Verification items for the finished model (mm, model axes). Give positions to 0.01 mm unless a question says otherwise; leave off trailing zeros. Order: outer loops, then holes, each group sorted by start corner. A loop starts at its lowest first (then second) coordinate and runs counter-clockwise, first axis right, second up.
(1) Scan lines: L1, parallel to Y at x = 102, z = 6 (3 decimals); L2, parallel to Y at x = 65, z = 2.25; L3, parallel to X at y = 166, z = 5.25 (3 decimals). Record each from-to range of solid material in increasing order.
(2) Sectioned sample at C-C on z = 3. Count the separate pieces of the cut face and the enclosed holes in it, plus the area to 3 significant figures.
(3) Sectioned sample at A-A on y = 185. Record the cut outline in (x, z).
(4) Gauge pin test, flat ends, axial feed: pin 1 (2 mm diameter, centred on y = 22.5, z = 3, fed in from +X); pin 2 (3 mm diameter, centred on x = -2.5, z = 2, fed in from -Y); pin 3 (1.5 mm diameter, centred on y = 225.5, z = 1.5, fed in from -X). Record the tip position at first contact, or that the pin passes through.
```python
from build123d import *

# Parameters (mm, degrees)
SKETCH2_W           = 6.096
SKETCH2_H           = 19.230769231
SKETCH2_W_2         = 19.230769231
SKETCH2_H_2         = 6.096
SKETCH2_W_3         = 19.23076923
SKETCH2_H_3         = 19.23076923
BOSS_EXTRUDE2_DEPTH = 6.096
SKETCH3_R           = 5
CUT_EXTRUDE1_DEPTH  = 363.225735762


with BuildPart() as part:
    # Sketch2 → Boss-Extrude2 (new body)
    # profile 1 of 29: a face of its own
    with BuildSketch(Plane.XY):
        Polygon((0, 19.230769231), (0, 0), (19.230769231, 0), (38.461538462, 0), (57.692307692, 0), (76.923076923, 0), (96.153846154, 0), (115.384615385, 0), (134.615384615, 0), (153.846153846, 0), (173.076923077, 0), (192.307692308, 0), (211.538461538, 0), (230.769230769, 0), (250, 0), (250, 19.230769231), (250, 38.461538462), (250, 57.692307692), (250, 76.923076923), (250, 96.153846154), (250, 115.384615385), (250, 134.615384615), (250, 153.846153846), (250, 173.076923077), (250, 192.307692308), (250, 211.538461538), (250, 230.769230769), (250, 250), (230.769230769, 250), (211.538461538, 250), (192.307692308, 250), (173.076923077, 250), (153.846153846, 250), (134.615384615, 250), (115.384615385, 250), (96.153846154, 250), (76.923076923, 250), (57.692307692, 250), (38.461538462, 250), (19.230769231, 250), (0, 250), (0, 230.769230769), (0, 211.538461538), (0, 192.307692308), (0, 173.076923077), (0, 153.846153846), (0, 134.615384615), (0, 115.384615385), (0, 96.153846154), (0, 76.923076923), (0, 57.692307692), (0, 38.461538462), align=None)
        Polygon((80.825, 104), (80.825, 80.825), (104, 80.825), (104, 77.65), (80.825, 77.65), (79.825, 77.65), (79.825, 80.825), (77.65, 80.825), (77.65, 104), align=None, mode=Mode.SUBTRACT)
        Polygon((146, 80.825), (169.175, 80.825), (169.175, 104), (172.35, 104), (172.35, 80.825), (170.175, 80.825), (170.175, 77.65), (169.175, 77.65), (146, 77.65), align=None, mode=Mode.SUBTRACT)
        Polygon((104, 169.175), (80.825, 169.175), (80.825, 146), (77.65, 146), (77.65, 169.175), (79.825, 169.175), (79.825, 172.35), (80.825, 172.35), (104, 172.35), align=None, mode=Mode.SUBTRACT)
        Polygon((169.175, 146), (169.175, 169.175), (146, 169.175), (146, 172.35), (169.175, 172.35), (170.175, 172.35), (170.175, 169.175), (172.35, 169.175), (172.35, 146), align=None, mode=Mode.SUBTRACT)
    # profile 2 of 29: a face of its own
    with BuildSketch(Plane.XY):
        with Locations((-3.048, 9.615384616)):
            Rectangle(SKETCH2_W, SKETCH2_H)
    # profile 3 of 29: a face of its own
    with BuildSketch(Plane.XY):
        with Locations((9.615384616, -3.048)):
            Rectangle(SKETCH2_W_2, SKETCH2_H_2)
    # profile 4 of 29: a face of its own
    with BuildSketch(Plane.XY):
        with Locations((48.076923077, -3.048)):
            Rectangle(SKETCH2_W_3, SKETCH2_H_2)
    # profile 5 of 29: a face of its own
    with BuildSketch(Plane.XY):
        with Locations((-3.048, 48.076923077)):
            Rectangle(SKETCH2_W, SKETCH2_H_3)
    # profile 6 of 29: a face of its own
    with BuildSketch(Plane.XY):
        with Locations((86.538461539, -3.048)):
            Rectangle(SKETCH2_W_2, SKETCH2_H_2)
    # profile 7 of 29: a face of its own
    with BuildSketch(Plane.XY):
        with Locations((-3.048, 86.538461539)):
            Rectangle(SKETCH2_W, SKETCH2_H)
    # profile 8 of 29: a face of its own
    with BuildSketch(Plane.XY):
        with Locations((125, -3.048)):
            Rectangle(SKETCH2_W_3, SKETCH2_H_2)
    # profile 9 of 29: a face of its own
    with BuildSketch(Plane.XY):
        with Locations((-3.048, 125)):
            Rectangle(SKETCH2_W, SKETCH2_H_3)
    # profile 10 of 29: a face of its own
    with BuildSketch(Plane.XY):
        with Locations((163.461538462, -3.048)):
            Rectangle(SKETCH2_W_2, SKETCH2_H_2)
    # profile 11 of 29: a face of its own
    with BuildSketch(Plane.XY):
        with Locations((-3.048, 163.461538462)):
            Rectangle(SKETCH2_W, SKETCH2_H)
    # profile 12 of 29: a face of its own
    with BuildSketch(Plane.XY):
        with Locations((201.923076923, -3.048)):
            Rectangle(SKETCH2_W_3, SKETCH2_H_2)
    # profile 13 of 29: a face of its own
    with BuildSketch(Plane.XY):
        with Locations((-3.048, 201.923076923)):
            Rectangle(SKETCH2_W, SKETCH2_H_3)
    # profile 14 of 29: a face of its own
    with BuildSketch(Plane.XY):
        with Locations((240.384615385, -3.048)):
            Rectangle(SKETCH2_W_2, SKETCH2_H_2)
    # profile 15 of 29: a face of its own
    with BuildSketch(Plane.XY):
        with Locations((-3.048, 240.384615385)):
            Rectangle(SKETCH2_W, SKETCH2_H)
    # profile 16 of 29: a face of its own
    with BuildSketch(Plane.XY):
        with Locations((253.048, 9.615384616)):
            Rectangle(SKETCH2_W, SKETCH2_H)
    # profile 17 of 29: a face of its own
    with BuildSketch(Plane.XY):
        with Locations((9.615384616, 253.048)):
            Rectangle(SKETCH2_W_2, SKETCH2_H_2)
    # profile 18 of 29: a face of its own
    with BuildSketch(Plane.XY):
        with Locations((253.048, 48.076923077)):
            Rectangle(SKETCH2_W, SKETCH2_H_3)
    # profile 19 of 29: a face of its own
    with BuildSketch(Plane.XY):
        with Locations((48.076923077, 253.048)):
            Rectangle(SKETCH2_W_3, SKETCH2_H_2)
    # profile 20 of 29: a face of its own
    with BuildSketch(Plane.XY):
        with Locations((253.048, 86.538461539)):
            Rectangle(SKETCH2_W, SKETCH2_H)
    # profile 21 of 29: a face of its own
    with BuildSketch(Plane.XY):
        with Locations((86.538461539, 253.048)):
            Rectangle(SKETCH2_W_2, SKETCH2_H_2)
    # profile 22 of 29: a face of its own
    with BuildSketch(Plane.XY):
        with Locations((253.048, 125)):
            Rectangle(SKETCH2_W, SKETCH2_H_3)
    # profile 23 of 29: a face of its own
    with BuildSketch(Plane.XY):
        with Locations((125, 253.048)):
            Rectangle(SKETCH2_W_3, SKETCH2_H_2)
    # profile 24 of 29: a face of its own
    with BuildSketch(Plane.XY):
        with Locations((253.048, 163.461538462)):
            Rectangle(SKETCH2_W, SKETCH2_H)
    # profile 25 of 29: a face of its own
    with BuildSketch(Plane.XY):
        with Locations((163.461538462, 253.048)):
            Rectangle(SKETCH2_W_2, SKETCH2_H_2)
    # profile 26 of 29: a face of its own
    with BuildSketch(Plane.XY):
        with Locations((253.048, 201.923076923)):
            Rectangle(SKETCH2_W, SKETCH2_H_3)
    # profile 27 of 29: a face of its own
    with BuildSketch(Plane.XY):
        with Locations((201.923076923, 253.048)):
            Rectangle(SKETCH2_W_3, SKETCH2_H_2)
    # profile 28 of 29: a face of its own
    with BuildSketch(Plane.XY):
        with Locations((253.048, 240.384615385)):
            Rectangle(SKETCH2_W, SKETCH2_H)
    # profile 29 of 29: a face of its own
    with BuildSketch(Plane.XY):
        with Locations((240.384615385, 253.048)):
            Rectangle(SKETCH2_W_2, SKETCH2_H_2)
    extrude(amount=BOSS_EXTRUDE2_DEPTH)

    # Sketch3 → Cut-Extrude1 (cut, through all)
    with BuildSketch(Plane(origin=(0, 0, 0), x_dir=(-1, 0, 0), z_dir=(0, 0, -1))):
        with Locations((-185, 185)):
            Circle(SKETCH3_R)
        with Locations((-65, 185)):
            Circle(SKETCH3_R)
        with Locations((-65, 65)):
            Circle(SKETCH3_R)
        with Locations((-185, 65)):
            Circle(SKETCH3_R)
    extrude(amount=-CUT_EXTRUDE1_DEPTH, mode=Mode.SUBTRACT)


solid = part.part
```
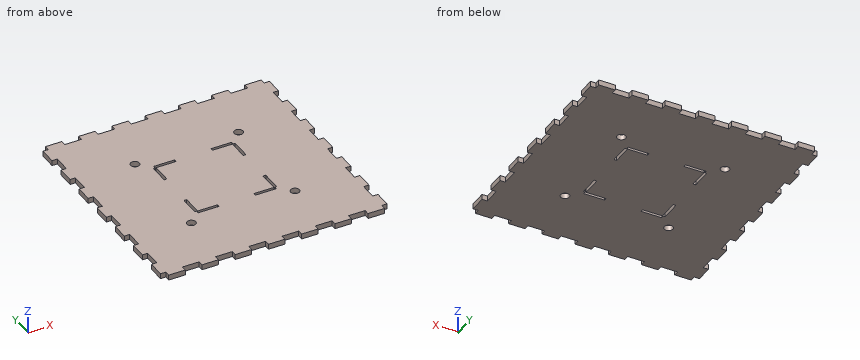
Ans:
1. L1: y = 0 to 77.65, 80.825 to 169.175, 172.35 to 250
1. L2: y = 0 to 60, 70 to 180, 190 to 250
1. L3: x = -6.096 to 77.65, 80.825 to 169.175, 172.35 to 256.096
2. separate pieces: 1
2. enclosed holes: 8
2. area: 64,900 mm2
3. outline: (0, 0) - (60, 0) - (60, 6.1) - (0, 6.1) - close; (70, 0) - (180, 0) - (180, 6.1) - (70, 6.1) - close; (190, 0) - (250, 0) - (250, 6.1) - (190, 6.1) - close
4. pin 1: stops at x = 250
4. pin 2: stops at y = 0
4. pin 3: stops at x = 0
